```python
from build123d import *

# Parameters (mm, degrees)
F1_DEPTH = 25


with BuildPart() as f1:
    # F0 (on Top) → F1 (new body)
    with BuildSketch(Plane.XY):
        with BuildLine():
            Line((39.599326, -61.959296), (39.599326, 32.040704))
            ThreePointArc((39.599326, 32.040704), (38.720646, 34.162024), (36.599326, 35.040704))
            Line((36.599326, 35.040704), (-17.400674, 35.040704))
            ThreePointArc((-17.400674, 35.040704), (-19.521995, 34.162024), (-20.400674, 32.040704))
            Line((-20.400674, 32.040704), (-20.400674, -61.959296))
            ThreePointArc((-20.400674, -61.959296), (-19.521995, -64.080617), (-17.400674, -64.959296))
            Line((-17.400674, -64.959296), (9.599326, -64.959296))
            Line((9.599326, -64.959296), (36.599326, -64.959296))
            ThreePointArc((36.599326, -64.959296), (38.720646, -64.080617), (39.599326, -61.959296))
        make_face()
        with BuildLine():
            Line((32.999326, -61.359296), (10.599326, -61.359296))
            Line((10.599326, -61.359296), (-12.800674, -61.359296))
            ThreePointArc((-12.800674, -61.359296), (-14.921995, -60.480617), (-15.800674, -58.359296))
            Line((-15.800674, -58.359296), (-15.800674, 28.440704))
            ThreePointArc((-15.800674, 28.440704), (-14.921995, 30.562024), (-12.800674, 31.440704))
            Line((-12.800674, 31.440704), (9.599326, 31.440704))
            Line((9.599326, 31.440704), (10.599326, 31.440704))
            Line((10.599326, 31.440704), (32.999326, 31.440704))
            ThreePointArc((32.999326, 31.440704), (35.120646, 30.562024), (35.999326, 28.440704))
            Line((35.999326, 28.440704), (35.999326, -58.359296))
            ThreePointArc((35.999326, -58.359296), (35.120646, -60.480617), (32.999326, -61.359296))
        make_face(mode=Mode.SUBTRACT)
    extrude(amount=F1_DEPTH)


solid = f1.part
```
Verification items for the finished model (mm, model axes). A direction names the side the tool comes from. Give positions to 0.01 mm unless a question says otherwise; leave off trailing zeros. Write each loop counter-clockwise with the first axis right and the second up, starting at its lowest first coordinate (ties: lowest second). Pieces come first, ordered by that corner, then holes. Notation, with made-up numbers: M -17,-6.5 L 21,-6.5 A11 ccw 21,-2.5 Z; hole C 35,28 d7. An arc over 180 degrees is marked long. One line per question, with ' | ' between items.
1) Section check B-B on x = -2. Enter the section's corners in (y, z).
Result:
outline: M -64.96,0 L -61.36,0 L -61.36,25 L -64.96,25 Z; M 31.44,0 L 35.04,0 L 35.04,25 L 31.44,25 Z
2) Mould release check, pull along Y, two halves, no side actions. Record for faces 3 (the cylindrical face through (35.1, -60.5, 12.3)), 4 (the cylindrical face through (-19.499, 34.185, 12.325)), 5 (the flat face through (-20.401, -14, 12)), 6 (the cylindrical face through (35.097, 30.585, 12.325)): released by +Y, released by -Y, zero draft, split by the parting line, or undercut.
Result:
face 3: undercut | face 4: released by +Y | face 5: zero draft | face 6: undercut
3) Set-up check for faces 1 (the cylindrical face through (-19.5, -64.1, 12.3)), 2 (the flat face through (10, -61.359, 12)): record each of +Z, -Z, +X, -X, +Y, -Y from which the full face is reachable in a straight line by a thin tool's end or side.
Result:
face 1: +Z, -Z, -X, -Y | face 2: +Z, -Z
4) Thickness scan on line 1 along Y through (x, z) = (21, 20.25); line 2 along X through (y, z) = (-27, 4.75). Record the ranges inside material, lowest first. Write a range as [from, to].
Result:
line 1: y = [-64.96, -61.36], [31.44, 35.04] | line 2: x = [-20.4, -15.8], [36, 39.6]
5) Section check A-A on y = 8. Enter the section's corners in (x, z).
Result:
outline: M -20.4,0 L -15.8,0 L -15.8,25 L -20.4,25 Z; M 36,0 L 39.6,0 L 39.6,25 L 36,25 Z
6) Section check C-C on z = 21. Enter the section's corners in (x, y).
Result:
outline: M -20.4,-61.96 A3 ccw -17.4,-64.96 L 36.6,-64.96 A3 ccw 39.6,-61.96 L 39.6,32.04 A3 ccw 36.6,35.04 L -17.4,35.04 A3 ccw -20.4,32.04 Z; hole M -15.8,-58.36 A3 ccw -12.8,-61.36 L 33,-61.36 A3 ccw 36,-58.36 L 36,28.44 A3 ccw 33,31.44 L -12.8,31.44 A3 ccw -15.8,28.44 Z
